Geometry check sheet. Reference: the model listing, model coordinates, mm. Give positions to 0.01 mm unless a question says otherwise; leave off trailing zeros. Order: outer loops, then holes, each group sorted by start corner. A loop starts at its lowest first (then second) coordinate and runs counter-clockwise, first axis right, second up. Notation, with made-up numbers: M 82,5.25 L 120,5.25 A12 cw 120,13.25 Z; hole C 30,72.5 d5. An arc over 180 degrees is marked long. Answer as a JSON object with one key per item and string values. Group by question number.
from build123d import *

# Parameters (mm, degrees)
BOSS_EXTRU_1_DEPTH = 1


with BuildPart() as part:
    # Esquisse4 → Boss.-Extru.1 (new body)
    with BuildSketch(Plane.XY):
        Polygon((109.153274168, 31.039696422), (109.153274168, 0.039696422), (132, 0.039696422), (137, 5.039696422), (137, 26.039696422), (132, 31.039696422), align=None)
        with BuildLine():
            Line((0, 4.039696422), (-22.5, 3.539696422))
            Line((-22.5, 3.539696422), (-22.5, 0.539696422))
            Line((-22.5, 0.539696422), (0, 0.039696422))
            Line((0, 0.039696422), (109.153274168, 0.039696422))
            Line((109.153274168, 0.039696422), (109.153274168, 31.039696422))
            Line((109.153274168, 31.039696422), (0, 31.039696422))
            Line((0, 31.039696422), (-35, 31.039696422))
            ThreePointArc((-35, 31.039696422), (-40.039696422, 26), (-35, 20.960303578))
            Line((-35, 20.960303578), (0, 20.960303578))
            ThreePointArc((0, 20.960303578), (0.041053045, 20.480151789), (0, 20))
            Line((0, 20), (-35, 20))
            ThreePointArc((-35, 20), (-37, 18), (-35, 16))
            Line((-35, 16), (0, 16))
            ThreePointArc((0, 16), (0.828427125, 14), (0, 12))
            Line((0, 12), (-22.5, 12))
            Line((-22.5, 12), (-22.5, 8))
            Line((-22.5, 8), (0, 8))
            ThreePointArc((0, 8), (0.808773964, 6.019848211), (0, 4.039696422))
        make_face()
        with BuildLine():
            ThreePointArc((-35, 17.1), (-35.9, 18), (-35, 18.9))
            Line((-35, 18.9), (-29, 18.9))
            ThreePointArc((-29, 18.9), (-28.1, 18), (-29, 17.1))
            Line((-29, 17.1), (-35, 17.1))
        make_face(mode=Mode.SUBTRACT)
        with BuildLine():
            ThreePointArc((-35, 25.1), (-35.9, 26), (-35, 26.9))
            Line((-35, 26.9), (-29, 26.9))
            ThreePointArc((-29, 26.9), (-28.1, 26), (-29, 25.1))
            Line((-29, 25.1), (-35, 25.1))
        make_face(mode=Mode.SUBTRACT)
        with BuildLine():
            Line((-35, 8), (-22.5, 8))
            Line((-22.5, 8), (-22.5, 12))
            Line((-22.5, 12), (-35, 12))
            ThreePointArc((-35, 12), (-37, 10), (-35, 8))
        make_face()
        with BuildLine():
            ThreePointArc((-35, 9.1), (-35.9, 10), (-35, 10.9))
            Line((-35, 10.9), (-29, 10.9))
            ThreePointArc((-29, 10.9), (-28.1, 10), (-29, 9.1))
            Line((-29, 9.1), (-35, 9.1))
        make_face(mode=Mode.SUBTRACT)
        with BuildLine():
            ThreePointArc((-35, 0.539696422), (-36.5, 2.039696422), (-35, 3.539696422))
            Line((-35, 3.539696422), (-22.5, 3.539696422))
            Line((-22.5, 3.539696422), (-22.5, 0.539696422))
            Line((-22.5, 0.539696422), (-35, 0.539696422))
        make_face()
        with BuildLine():
            ThreePointArc((-29, 1.139696422), (-28.1, 2.039696422), (-29, 2.939696422))
            Line((-29, 2.939696422), (-35, 2.939696422))
            ThreePointArc((-35, 2.939696422), (-35.9, 2.039696422), (-35, 1.139696422))
            Line((-35, 1.139696422), (-29, 1.139696422))
        make_face(mode=Mode.SUBTRACT)
    extrude(amount=BOSS_EXTRU_1_DEPTH)


solid = part.part
1. Depth check by flat-ended pin: pin 1 (0.5 mm diameter, centred on x = -32, z = 0.5, fed in from -Y). Enter the tip coordinate at first touch or a pass-through.
2. Cross-section at B-B (z = 0.15). State how many separate pieces and enclosed holes the cut face has, and give its area (3 significant figures).
3. Cross-section at A-A (x = -7.5). Record the cut outline in (y, z).
4. Thickness scan on line 1 along Y through (x, z) = (-23.5, 0.2); line 2 along X through (y, z) = (6, 0.7); line 3 along X through (y, z) = (26.5, 0.95). Record the ranges inside material, lowest first. Write a range as [from, to].
Report:
{
 "1": {"pin 1": "stops at y = 0.54"},
 "2": {"separate pieces": "1", "enclosed holes": "4", "area": "4,970 mm2"},
 "3": {"outline": "M 0.21,0 L 3.87,0 L 3.87,1 L 0.21,1 Z; M 8,0 L 12,0 L 12,1 L 8,1 Z; M 16,0 L 20,0 L 20,1 L 16,1 Z; M 20.96,0 L 31.04,0 L 31.04,1 L 20.96,1 Z"},
 "4": {"line 1": "y = [0.54, 3.54], [8, 12], [16, 20], [20.96, 31.04]", "line 2": "x = [0.81, 137]", "line 3": "x = [-40.01, -35.75], [-28.25, 136.54]"}
}
